Print and shaded views of the part. All mm, measured from the part's lowest x, y and z. Give positions to 0.01 mm unless a question says otherwise; leave off trailing zeros. Loops run counter-clockwise (first coordinate to the right, second up) from the corner with the lowest first, then second, coordinate; pieces in that order, holes last. Notation, with made-up numbers: (85.25, 53.5) - (108.25, 53.5) arc R20 ccw to (108.25, 57.5) - close; hole circle Ø5 at (49.25, 29). An arc over 180 degrees is marked (long way). Return JSON: item names as keys, results as strings.
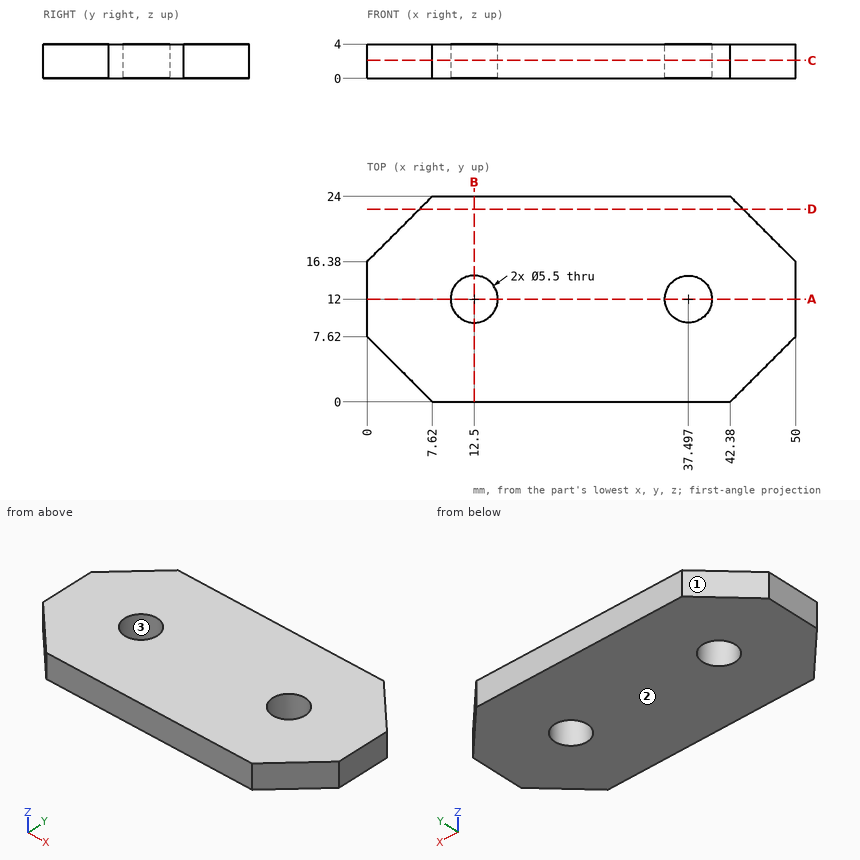
1. Cut at D-D, the plane y = 22.5. Write the cut outline in (x, z).
Values follow:
{"outline": "(6.12, 0) - (43.88, 0) - (43.88, 4) - (6.12, 4) - close"}
2. Cut at C-C, the plane z = 2.1. Write the cut outline in (x, y), plus the area to 3 significant figures.
Values follow:
{"outline": "(0, 7.62) - (7.62, 0) - (42.38, 0) - (50, 7.62) - (50, 16.38) - (42.38, 24) - (7.62, 24) - (0, 16.38) - close; hole circle Ø5.5 at (12.5, 12); hole circle Ø5.5 at (37.5, 12)", "area": "1,040 mm²"}
3. Pull direction Y, two halves, no side cores. Call the marked faces 1, 2 and 3: +Y half, -Y half, draft (parallel to the pull), parting line (faces both ways), or undercut.
Values follow:
{"face 1": "+Y half", "face 2": "draft", "face 3": "undercut"}
4. Drop flat-ended pins along their axis: P1, Ø1, axis at y = 19.5, z = 2, coming from the +X side; P2, Ø1.5, axis at y = 17, z = 3.5, coming from the -X side. Give the stop position or say it passes through.
Values follow:
{"P1": "stops at x = 47.38", "P2": "stops at x = 0"}
5. Cut at A-A, the plane y = 12. Write the cut outline in (x, z).
Values follow:
{"outline": "(0, 0) - (9.75, 0) - (9.75, 4) - (0, 4) - close; (15.25, 0) - (34.75, 0) - (34.75, 4) - (15.25, 4) - close; (40.25, 0) - (50, 0) - (50, 4) - (40.25, 4) - close"}
6. Cut at B-B, the plane x = 12.5. Write the cut outline in (y, z), plus the area to 3 significant figures.
Values follow:
{"outline": "(0, 0) - (9.25, 0) - (9.25, 4) - (0, 4) - close; (14.75, 0) - (24, 0) - (24, 4) - (14.75, 4) - close", "area": "74.0 mm²"}
7. Drill centre lines: probe 1 along Y at (x, z) = (12.5, 1.8); probe 2 along X at (y, z) = (10.5, 1.75) (1 decimal); probe 3 along X at (y, z) = (9.75, 2.2) (1 decimal). Where is each one in solid material? Low to high.
Values follow:
{"probe 1": "y = 0 to 9.25, 14.75 to 24", "probe 2": "x = 0 to 10.2, 14.8 to 35.2, 39.8 to 50", "probe 3": "x = 0 to 10.9, 14.1 to 35.9, 39.1 to 50"}
